```python
from build123d import *

# Parameters (mm, degrees)
SKETCH2_W             = 33.5
SKETCH2_H             = 33.5
BOSS_EXTRUDE1_DEPTH   = 2
M4_TAPPED_HOLE1_DEPTH = 2


# Read off the part's stored shape, not the designer's step: M4 Tapped Hole1
with BuildPart() as part:
    # Sketch2 → Boss-Extrude1 (new body)
    with BuildSketch(Plane(origin=(0, 0, 0), x_dir=(1, 0, 0), z_dir=(0, 1, 0))):
        Rectangle(SKETCH2_W, SKETCH2_H)
    extrude(amount=BOSS_EXTRUDE1_DEPTH)

    # M4 Tapped Hole1 outline → M4 Tapped Hole1 (cut)
    with BuildSketch(Plane(origin=(0, 0, 0), x_dir=(1, 0, 0), z_dir=(0, 1, 0))):
        with BuildLine():
            Line((16.75, -16.75), (16.75, -14.562613646))
            ThreePointArc((16.75, -14.562613646), (14.083273811, -14.083273811), (14.562613646, -16.75))
            Line((14.562613646, -16.75), (16.75, -16.75))
        make_face()
        with BuildLine():
            ThreePointArc((14.562613646, 16.75), (14.083273811, 14.083273811), (16.75, 14.562613646))
            Line((16.75, 14.562613646), (16.75, 16.75))
            Line((16.75, 16.75), (14.562613646, 16.75))
        make_face()
        with BuildLine():
            Line((-16.75, -16.75), (-14.562613646, -16.75))
            ThreePointArc((-14.562613646, -16.75), (-14.083273811, -14.083273811), (-16.75, -14.562613646))
            Line((-16.75, -14.562613646), (-16.75, -16.75))
        make_face()
        with BuildLine():
            ThreePointArc((-16.75, 14.562613646), (-14.083273811, 14.083273811), (-14.562613646, 16.75))
            Line((-14.562613646, 16.75), (-16.75, 16.75))
            Line((-16.75, 16.75), (-16.75, 14.562613646))
        make_face()
    extrude(amount=M4_TAPPED_HOLE1_DEPTH, mode=Mode.SUBTRACT)


solid = part.part
```
Input: part model. Units: mm. Frame: model coordinates. Give positions to 0.01 mm unless a question says otherwise; leave off trailing zeros. Order: outer loops, then holes, each group sorted by start corner. A loop starts at its lowest first (then second) coordinate and runs counter-clockwise, first axis right, second up.
1. Line query: probe 1 along Z at (x, y) = (-15.25, 0.5). Output: solid intervals per line, ascending.
Computed:
probe 1: z = -13.6 to 13.6
2. Draft query along Z for faces 1 (the face through (14.05, 0.99, -14.12)), 2 (the face through (-16.75, 1, 0)), 3 (the face through (-14.05, 0.99, 14.12)), 4 (the face through (0, 1, 16.75)). Return one class per face: released by +Z, released by -Z, zero draft, split by the parting line, or undercut.
Computed:
face 1: undercut
face 2: zero draft
face 3: undercut
face 4: released by +Z
3. Cut plane B-B (z = -15.25). Return loops of the section in (x, y), and give its area (3 significant figures).
Computed:
outline: (-13.6, 0) - (13.6, 0) - (13.6, 2) - (-13.6, 2) - close
area: 54.4 mm2
4. Cut plane A-A (y = 0.75). Return loops of the section in (x, z).
Computed:
outline: (-16.75, -14.56) arc R1.65 cw (long way) to (-14.56, -16.75) - (14.56, -16.75) arc R1.65 cw (long way) to (16.75, -14.56) - (16.75, 14.56) arc R1.65 cw (long way) to (14.56, 16.75) - (-14.56, 16.75) arc R1.65 cw (long way) to (-16.75, 14.56) - close
5. Cut plane C-C (x = 15.25). Return loops of the section in (y, z).
Computed:
outline: (0, -13.6) - (2, -13.6) - (2, 13.6) - (0, 13.6) - close
